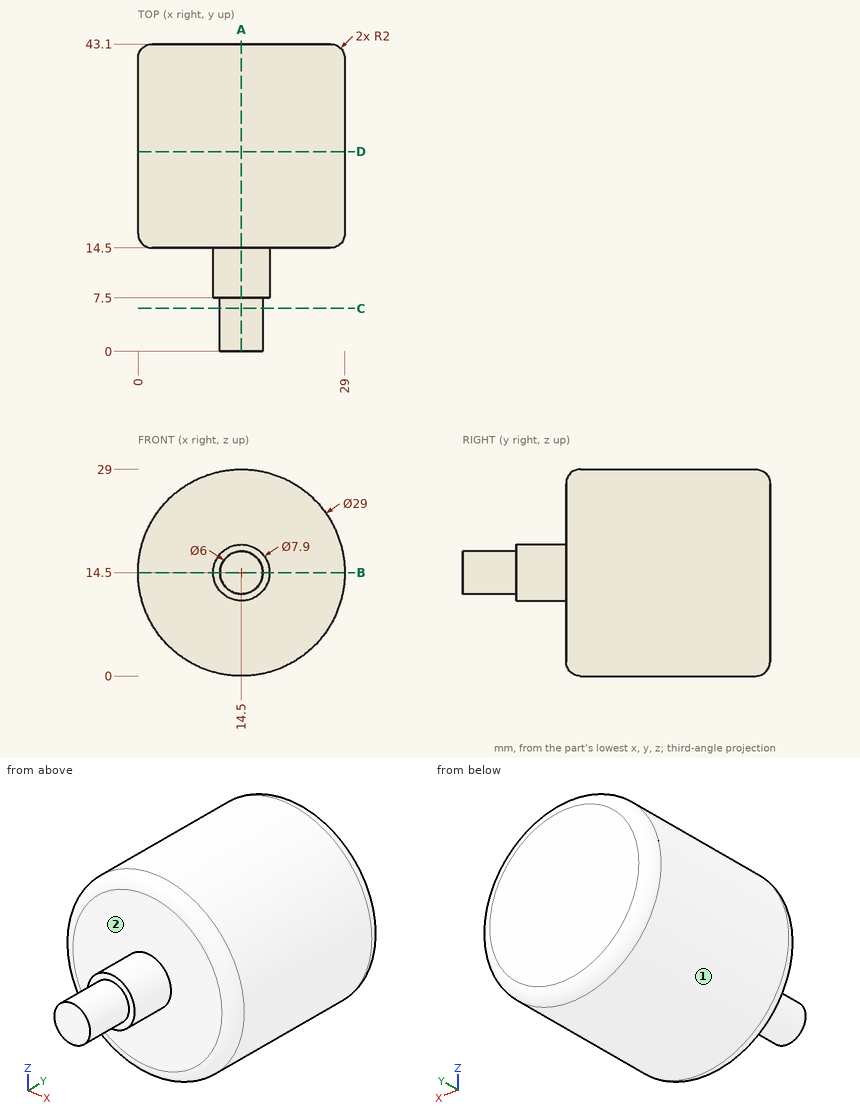
Could you check a few things on this drawing? It's one solid part, dimensions in mm from its lowest x, y, z. A direction names the side the tool comes from. Give positions to 0.01 mm unless a question says otherwise; leave off trailing zeros. Write each loop counter-clockwise with the first axis right and the second up, starting at its lowest first coordinate (ties: lowest second). Pieces come first, ordered by that corner, then holes. Notation, with made-up numbers: (-14, 27.25) -> (23, 27.25) arc R31 ccw to (23, 55.25) -> close; hole circle Ø3 at (10.25, 31.25). An arc over 180 degrees is marked (long way). Answer as a JSON object with one key per item and string values.
Q1. Which directions (+Z, -Z, +X, -X, +Y, -Y) give clear straight access to the entire face, cutting with the end or side of a thin tool? Please do the marked faces 1 and 2.
Taken from the geometry:
{"face 1": "+Y, -Y", "face 2": "-Y"}
Q2. Suppose I cut it at C-C on y = 6. Write out the boundary of the cut face in (x, z), then the cut area to 3 significant figures.
Taken from the geometry:
{"outline": "circle Ø6 at (14.5, 14.5)", "area": "28.3 mm²"}
Q3. Suppose I cut it at A-A on x = 14.5. Write out the boundary of the cut face in (y, z).
Taken from the geometry:
{"outline": "(0, 11.5) -> (7.5, 11.5) -> (7.5, 10.55) -> (14.5, 10.55) -> (14.5, 2) arc R2 ccw to (16.5, 0) -> (41.1, 0) arc R2 ccw to (43.1, 2) -> (43.1, 27) arc R2 ccw to (41.1, 29) -> (16.5, 29) arc R2 ccw to (14.5, 27) -> (14.5, 18.45) -> (7.5, 18.45) -> (7.5, 17.5) -> (0, 17.5) -> close"}
Q4. Please list where these lines run through material, in increasing order: L1, parallel to Y at x = 13, z = 20.75; L2, parallel to Y at x = 15.5, z = 11.5; L3, parallel to X at y = 28, z = 21.5.
Taken from the geometry:
{"L1": "y = 14.5 to 43.1", "L2": "y = 7.5 to 43.1", "L3": "x = 1.8 to 27.2"}
Q5. Will these pins go through, and if not, where does the flat tip stop? pin 1 Ø2 at (x, y) = (10, 24) entering from +Z; pin 2 Ø2 at (x, z) = (7.5, 21.5) entering from -Y.
Taken from the geometry:
{"pin 1": "stops at z = 28.57", "pin 2": "stops at y = 14.5"}
Q6. Suppose I cut it at B-B on z = 14.5. Write out the boundary of the cut face in (x, y).
Taken from the geometry:
{"outline": "(0, 16.5) arc R2 ccw to (2, 14.5) -> (10.55, 14.5) -> (10.55, 7.5) -> (11.5, 7.5) -> (11.5, 0) -> (17.5, 0) -> (17.5, 7.5) -> (18.45, 7.5) -> (18.45, 14.5) -> (27, 14.5) arc R2 ccw to (29, 16.5) -> (29, 41.1) arc R2 ccw to (27, 43.1) -> (2, 43.1) arc R2 ccw to (0, 41.1) -> close"}
Q7. Suppose I cut it at D-D on y = 28. Write out the boundary of the cut face in (x, z), then the cut area to 3 significant figures.
Taken from the geometry:
{"outline": "circle Ø29 at (14.5, 14.5)", "area": "661 mm²"}
